Work out the finished part from the listing and answer in its coordinate system (mm). Round coordinates to 2 decimals unless told otherwise and drop trailing zeros. Return JSON: item names as keys, results as strings.
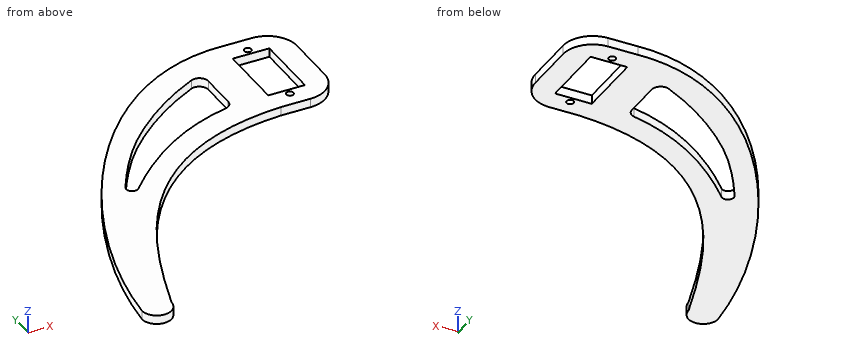
from build123d import *

# Parameters (mm, degrees)
SKETCH_R    = 1.2
SKETCH_W    = 12.4
SKETCH_H    = 23
PAD_DEPTH   = 3
FILLET_R    = 10
FILLET001_R = 3


with BuildPart() as part:
    # Sketch → Pad (new body)
    with BuildSketch(Plane.XY):
        with BuildLine():
            add(Edge.make_bspline(
                [(-95, -100), (-90.935824, -49.378152), (-52.268879, 20.279381), (-5.815751, 19)],
                knots=[0, 0, 0, 0, 1, 1, 1, 1], degree=3, weights=[6, 5.94, 6, 6]))
            Line((-5.815751, 19), (14.184249, 19))
            Line((14.184249, 19), (14.184249, -19))
            Line((14.184249, -19), (-5.815751, -19))
            add(Edge.make_bspline(
                [(-85, -100), (-74.069861, -64.186531), (-57.431784, -21.648657), (-5.815751, -19)],
                knots=[0, 0, 0, 0, 1, 1, 1, 1], degree=3))
            ThreePointArc((-85, -100), (-90, -105), (-95, -100))
        make_face()
        with Locations((0, 13.62)):
            Circle(SKETCH_R, mode=Mode.SUBTRACT)
        with Locations((0, -13.62)):
            Circle(SKETCH_R, mode=Mode.SUBTRACT)
        Rectangle(SKETCH_W, SKETCH_H, mode=Mode.SUBTRACT)
        with BuildLine():
            Line((-18.437941, 8.511872), (-18.437941, -11.5))
            add(Edge.make_bspline(
                [(-18.437941, -11.5), (-34.8974, -14.6095), (-49.1502, -22.8021), (-64.391878, -39.189094)],
                knots=[0, 0, 0, 0, 1, 1, 1, 1], degree=3))
            ThreePointArc((-64.391878, -39.189094), (-67.189094, -39.608122), (-67.608122, -36.810906))
            add(Edge.make_bspline(
                [(-18.437941, 8.511872), (-29.646872, 3.697302), (-46.497875, -7.962993), (-59.361809, -22.256252), (-67.608122, -36.810906)],
                knots=[0, 0, 0, 0, 0.5, 1, 1, 1, 1], degree=3))
        make_face(mode=Mode.SUBTRACT)
    extrude(amount=PAD_DEPTH)

    # Fillet
    fillet_edges = [part.edges().sort_by_distance(p)[0] for p in [
        (14.184249, -19, 1.5),
        (14.184249, 19, 1.5),
    ]]
    fillet(fillet_edges, radius=FILLET_R)

    # Fillet001
    fillet001_edges = [part.edges().sort_by_distance(p)[0] for p in [
        (-18.437941, 8.511872, 1.5),
        (-18.437941, -11.5, 1.5),
    ]]
    fillet(fillet001_edges, radius=FILLET001_R)


solid = part.part
1) Find the intervals of material crossed by L1, parallel to Y at x = 0, z = 2.3; L2, parallel to X at y = -8.5, z = 2.6; L3, parallel to X at y = 5.5, z = 1, in increasing order.
Verdict:
{"L1": "y = -19 to -14.82, -12.42 to -11.5, 11.5 to 12.42, 14.82 to 19", "L2": "x = -56.75 to -45.36, -18.44 to -6.2, 6.2 to 14.18", "L3": "x = -42.28 to -24.85, -18.93 to -6.2, 6.2 to 14.18"}
2) Section A-A (z = 2) is taken. Count the separate pieces of the cut face and the enclosed holes in it, and give its area (3 significant figures).
Verdict:
{"separate pieces": "1", "enclosed holes": "4", "area": "2,920 mm2"}
3) Flat-ended cylindrical pins translate along their axes: pin 1 (1.5 mm diameter, centred on y = -34.5, z = 2.5, fed in from -X); pin 2 (1.5 mm diameter, centred on x = -2.5, z = 1, fed in from +Y); pin 3 (1.5 mm diameter, centred on x = -1.5, z = 2, fed in from -Y). Find the tip coordinate at first contact, or state that the pin passes through.
Verdict:
{"pin 1": "stops at x = -74.86", "pin 2": "stops at y = 19", "pin 3": "stops at y = -19"}
